Design review of the part built by this model. Coordinates are the model's own, in mm. Face numbers are marked on the shaded views. Coordinates: 2 decimals unless noted, no trailing zeros. Write each loop counter-clockwise with the first axis right and the second up, starting at its lowest first coordinate (ties: lowest second). Pieces come first, ordered by that corner, then holes.
Q1. Add section A-A, the plane y = -39. Give the boundary of the cut face in (x, z), plus the area to 3 significant figures.
Q2. Clearance check with flat-ended pins moving along their axes: pin 1 Ø1 at (y, z) = (-10, -13) entering from +X; pin 2 Ø13 at (x, y) = (6, -6.5) entering from +Z; pin 3 Ø4 at (y, z) = (-53.5, -70) entering from -X. State where each tip first meets the part, or that it passes through.
Q3. The part is to be moulded in two halves that separate along Z. For the marked faces 1, 2 and 3, say which applies: +Z half, -Z half, draft (parallel to the pull), parting line (faces both ways), or undercut.
Q4. To check wall thickness, follow probe 1 along Z at (x, y) = (0, -35.65); probe 2 along Y at (x, z) = (0, -18.5); probe 3 along Y at (x, z) = (0, -29.7). State the ranges of each line that lie inside material, in increasing order.
Q5. Add section B-B, the plane z = -7.5. Give the boundary of the cut face in (x, y), plus the area to 3 significant figures.
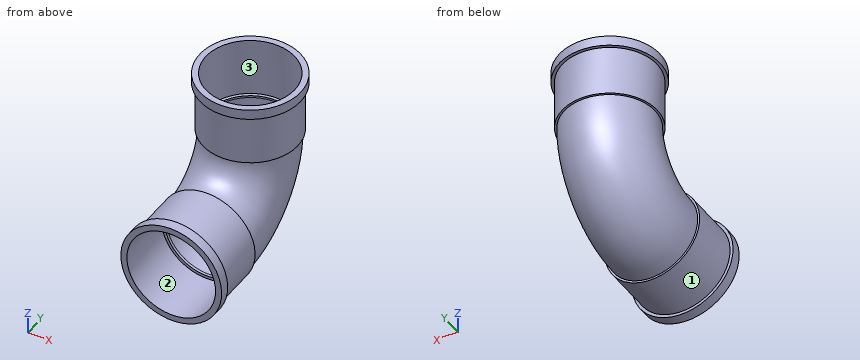
from build123d import *

# Parameters (mm, degrees)
SKELETON_R           = 23.5
SKELETON_R_2         = 22
SKELETON_R_3         = 20.5
BOSS_EXTRUDE1_DEPTH  = 30
SKELETON_3_R         = 22
SKELETON_3_R_2       = 20.5
CUT_EXTRUDE1_DEPTH   = 29
BOSS_EXTRUDE3_START  = -65
SKETCH6_R            = 23.5
SKETCH6_R_2          = 20.5
BOSS_EXTRUDE3_DEPTH  = 30
CUT_EXTRUDE2_START   = -65
SKETCH6_5_R          = 22
CUT_EXTRUDE2_DEPTH   = 29
SWEEP1_PROFILE_R     = 22.5
CUT_SWEEP1_PROFILE_R = 20.5
SKETCH36_W           = 5
SKETCH36_H           = 1.5
SKETCH36_3_W         = 1.5
SKETCH36_3_H         = 5


with BuildPart() as part:
    # Skeleton → Boss-Extrude1 (new body)
    # profile 1 of 2: a face of its own
    with BuildSketch(Plane.XY):
        Circle(SKELETON_R)
        Circle(SKELETON_R_2, mode=Mode.SUBTRACT)
    # profile 2 of 2: a face of its own
    with BuildSketch(Plane.XY):
        Circle(SKELETON_R_2)
        Circle(SKELETON_R_3, mode=Mode.SUBTRACT)
    extrude(amount=-BOSS_EXTRUDE1_DEPTH)

    # Skeleton<3> → Cut-Extrude1 (cut)
    with BuildSketch(Plane.XY):
        Circle(SKELETON_3_R)
        Circle(SKELETON_3_R_2, mode=Mode.SUBTRACT)
    extrude(amount=-CUT_EXTRUDE1_DEPTH, mode=Mode.SUBTRACT)



with BuildPart() as body_2:
    # Sketch6 → Boss-Extrude3 (new body)
    with BuildSketch(Plane(origin=(0, 0, 0), x_dir=(1, 0, 0), z_dir=(0, 1, 0)).offset(BOSS_EXTRUDE3_START)):
        with Locations(Location((0, 65, 0), (0, 0, 270))):
            Circle(SKETCH6_R)
        with Locations(Location((0, 65, 0), (0, 0, 270))):
            Circle(SKETCH6_R_2, mode=Mode.SUBTRACT)
    extrude(amount=BOSS_EXTRUDE3_DEPTH)

    # Sketch6<5> → Cut-Extrude2 (cut)
    with BuildSketch(Plane(origin=(0, 0, 0), x_dir=(1, 0, 0), z_dir=(0, 1, 0)).offset(CUT_EXTRUDE2_START)):
        with Locations(Location((0, 65, 0), (0, 0, 90))):
            Circle(SKETCH6_5_R)
    extrude(amount=CUT_EXTRUDE2_DEPTH, mode=Mode.SUBTRACT)


with BuildPart() as part_1:
    add(part.part)

    add(body_2.part)  # Sweep1 merges body 2
    # Sweep1: sweep along a path in Sketch4
    with BuildLine(Plane(origin=(0, 0, 0), x_dir=(0, 0, -1), z_dir=(1, 0, 0))) as sweep1_path:
        Line((29.074908745, 0), (30, 0))
        ThreePointArc((30, 0), (54.748737342, -10.251262658), (65, -35))
        Line((65, -35), (65, -36.362694274))
    # Sweep1 profile (on start of the path) → Sweep1 (sweep)
    with BuildSketch(Plane(origin=(0, 0, -29.074908745), x_dir=(-1, 0, 0), z_dir=(0, 0, -1))):
        Circle(SWEEP1_PROFILE_R)
    sweep(path=sweep1_path.line)

    # Cut-Sweep1: sweep along a path in Sketch4<2>
    with BuildLine(Plane(origin=(0, 0, 0), x_dir=(0, 0, -1), z_dir=(1, 0, 0))) as cut_sweep1_path:
        Line((29.074908745, 0), (30, 0))
        ThreePointArc((30, 0), (54.748737342, -10.251262658), (65, -35))
        Line((65, -35), (65, -36.362694274))
    # Cut-Sweep1 profile (on start of the path) → Cut-Sweep1 (sweep, cut)
    with BuildSketch(Plane(origin=(0, 0, -29.074908745), x_dir=(-1, 0, 0), z_dir=(0, 0, -1))):
        Circle(CUT_SWEEP1_PROFILE_R)
    sweep(path=cut_sweep1_path.line, mode=Mode.SUBTRACT)

    # Sketch36 → Revolve1 (revolve)
    with BuildSketch(Plane(origin=(0, 0, 0), x_dir=(0, 0, -1), z_dir=(1, 0, 0)), mode=Mode.PRIVATE) as revolve1_sk:
        with Locations((2.5, 24.25)):
            Rectangle(SKETCH36_W, SKETCH36_H)
    revolve(revolve1_sk.sketch.rotate(Axis((0, 0, 0), (0, 0, -1)), 90), axis=Axis((0, 0, 0), (0, 0, -1)))

    # Sketch36<3> → Revolve2 (revolve)
    with BuildSketch(Plane(origin=(0, 0, 0), x_dir=(0, 0, -1), z_dir=(1, 0, 0)), mode=Mode.PRIVATE) as revolve2_sk:
        with Locations((89.25, -62.5)):
            Rectangle(SKETCH36_3_W, SKETCH36_3_H)
    revolve(revolve2_sk.sketch.rotate(Axis((0, 0, -65), (0, -1, 0)), 180), axis=Axis((0, 0, -65), (0, -1, 0)))


solid = part_1.part
Here are the results:
1. outline: circle Ø47 at (0, -65); hole circle Ø44 at (0, -65)
1. area: 214 mm2
2. pin 1: stops at x = 21.49
2. pin 2: stops at z = -70.81
2. pin 3: stops at x = -23.31
3. face 1: parting line
3. face 2: undercut
3. face 3: draft
4. probe 1: z = -88.5 to -85.5, -44.5 to -41.5
4. probe 2: y = -23.5 to -22, 22 to 23.5
4. probe 3: y = -23.5 to -20.5, 20.5 to 23.5
5. outline: circle Ø47 at (0, 0); hole circle Ø44 at (0, 0)
5. area: 214 mm2
